Verification items for this drawing (mm, ordinates from the low corner). A direction names the side the tool comes from. Round coordinates to 2 decimals unless told otherwise and drop trailing zeros. Order: outer loops, then holes, each group sorted by start corner. A loop starts at its lowest first (then second) coordinate and runs counter-clockwise, first axis right, second up. Notation, with made-up numbers: (-1.5, 75) -> (11.5, 75) arc R21 ccw to (11.5, 88) -> close; hole circle Ø3 at (25.25, 16.5). An arc over 180 degrees is marked (long way). Return JSON: item names as keys, results as strings. Group by question number.
Item 1: Depth check by flat-ended pin: pin 1 Ø1 at (x, y) = (140, 90) entering from -Z (1 decimal); pin 2 Ø10 at (x, y) = (578, 154.5) entering from +Z. Enter the tip coordinate at first touch or a pass-through.
Item 2: Sectioned sample at D-D on z = 150. Record the cut outline in (x, y), plus the area to 3 significant figures.
Item 3: Draft check along X on the marked faces 1, 2 and 3. Enter one of: pulls with the +X half, pulls with the -X half, needs draft (parallel to the pull), parting line crosses it, or undercut.
Item 4: Sectioned sample at C-C on x = 545. Record the cut outline in (y, z).
Item 5: Sectioned sample at A-A on z = 460. Record the cut outline in (x, y), plus the area to 3 significant figures.
Item 6: Sectioned sample at B-B on y = 95.5. Record the cut outline in (x, z).
Item 7: Scan lines: probe 1 along X at (y, z) = (190, 516); probe 2 along Z at (x, y) = (579.5, 57); probe 3 along X at (y, z) = (17, 44.5) (1 decimal). Record each from-to range of solid material in increasing order. Write a range as from..to.
Item 8: Access from +Z, -Z, +X, -X, +Y, -Y to the whole of each face (thin tool, end or side, straight path). Record for the marked faces 4 and 5.
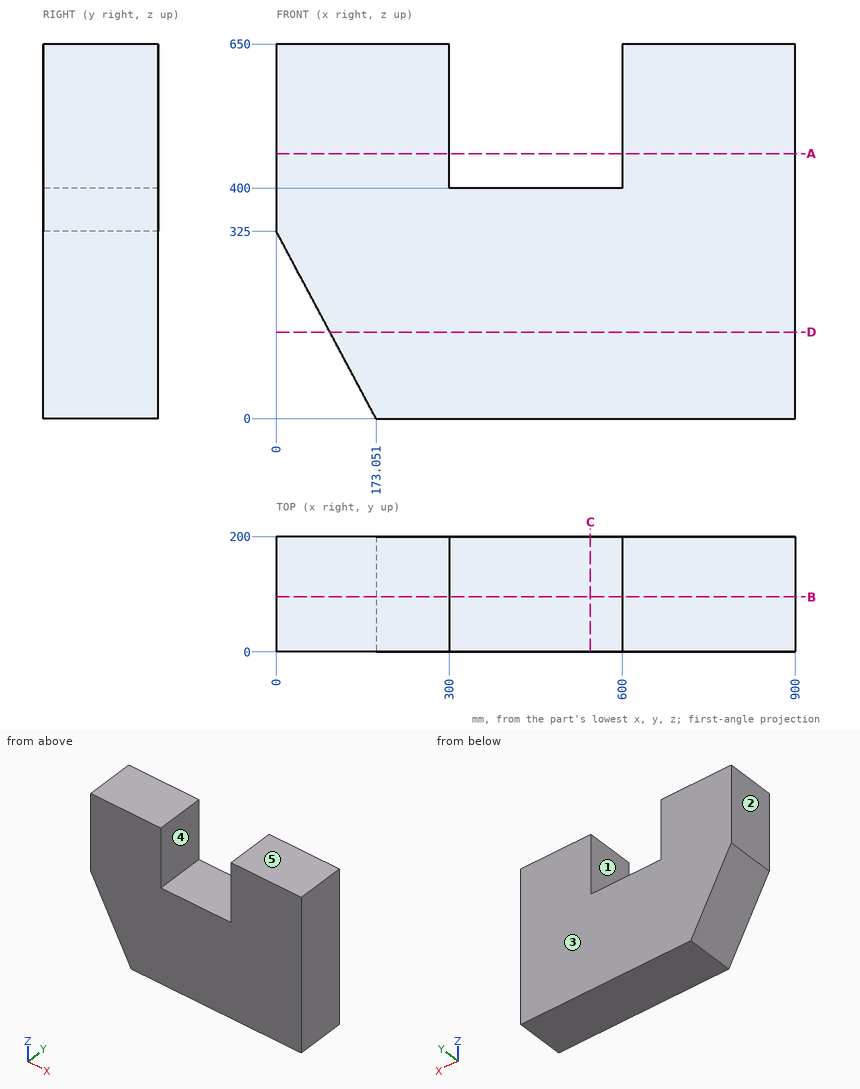
Recorded:
{
 "1": {"pin 1": "z = 61.1", "pin 2": "z = 400"},
 "2": {"outline": "(93.18, 0) -> (900, 0) -> (900, 200) -> (93.18, 200) -> close", "area": "161,000 mm²"},
 "3": {"face 1": "undercut", "face 2": "pulls with the -X half", "face 3": "needs draft"},
 "4": {"outline": "(0, 0) -> (200, 0) -> (200, 400) -> (0, 400) -> close"},
 "5": {"outline": "(0, 0) -> (300, 0) -> (300, 200) -> (0, 200) -> close; (600, 0) -> (900, 0) -> (900, 200) -> (600, 200) -> close", "area": "120,000 mm²"},
 "6": {"outline": "(0, 325) -> (173.05, 0) -> (900, 0) -> (900, 650) -> (600, 650) -> (600, 400) -> (300, 400) -> (300, 650) -> (0, 650) -> close"},
 "7": {"probe 1": "0..300, 600..900", "probe 2": "0..400", "probe 3": "149.4..900"},
 "8": {"face 4": "+Z, +Y, -Y", "face 5": "+Z, +X, -X, +Y, -Y"}
}
